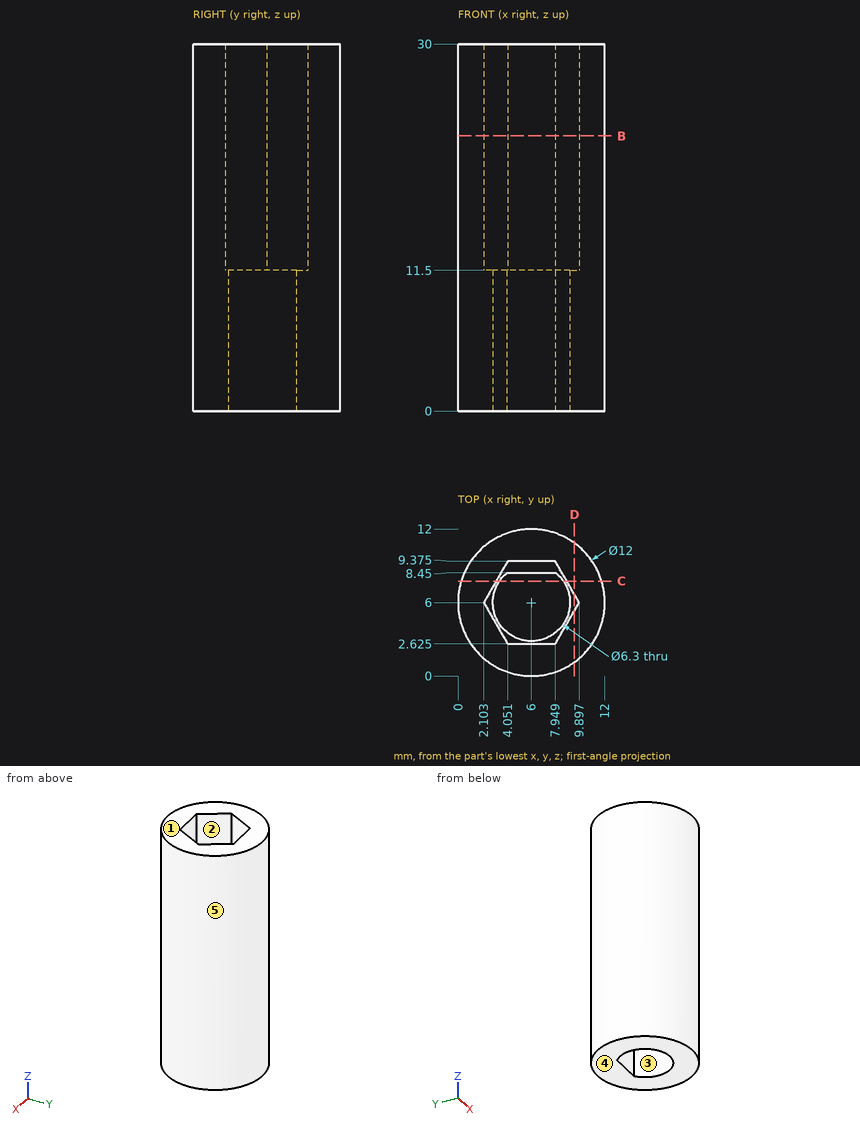
Verification items for this drawing (mm, ordinates from the low corner). A direction names the side the tool comes from. Coordinates: 2 decimals unless noted, no trailing zeros. Write each loop counter-clockwise with the first axis right and the second up, starting at its lowest first coordinate (ties: lowest second). Pieces come first, ordered by that corner, then holes. Notation, with made-up numbers: M -32,42.5 L -22,42.5 A23 cw -22,80.5 Z; hole C 68.5,54 d9. An arc over 180 degrees is marked long. Use CSV: the item, a comma, the result in double quotes.
Q1. Set-up check for the marked faces 1 and 2: record each of +Z, -Z, +X, -X, +Y, -Y from which the full face is reachable in a straight line by a thin tool's end or side.
Computed values:
face 1,"+Z, +X, -X, +Y, -Y"
face 2,"+Z"
Q2. Go/stop test with flat-tipped pins: P1, Ø4.5, axis at x = 5.5, z = 22, coming from the +Y side; P2, Ø5, axis at x = 10.5, z = 24.5, coming from the +Y side; P3, Ø1, axis at x = 3.5, z = 9.5, coming from the -Y side. Record where each tip stops, or that it passes through.
Computed values:
P1,"y = 12"
P2,"y = 11.66"
P3,"y = 0.34"
Q3. Section check B-B, the plane z = 22.5. Enter the section's corners in (x, y) (1 decimal).
Computed values:
outline,"C 6,6 d12; hole M 2.1,6 L 4.1,2.6 L 7.9,2.6 L 9.9,6 L 7.9,9.4 L 4.1,9.4 Z"
Q4. Section check C-C, the plane y = 7.75. Enter the section's corners in (x, z).
Computed values:
outline,"M 0.26,0 L 3.38,0 L 3.38,11.5 L 3.11,11.5 L 3.11,30 L 0.26,30 Z; M 8.62,0 L 11.74,0 L 11.74,30 L 8.89,30 L 8.89,11.5 L 8.62,11.5 Z"
Q5. Thickness scan on line 1 along Y through (x, z) = (6, 27.5) (1 decimal); line 2 along Y through (x, z) = (6, 6.5); line 3 along X through (y, z) = (7.75, 10.75). Record the ranges inside material, lowest first. Write a range as [from, to].
Computed values:
line 1,"[0, 2.6], [9.4, 12]"
line 2,"[0, 2.85], [8.45, 12]"
line 3,"[0.26, 3.38], [8.62, 11.74]"
Q6. Section check D-D, the plane x = 9.5. Enter the section's corners in (y, z), and give its area (3 significant figures).
Computed values:
outline,"M 1.13,0 L 10.87,0 L 10.87,30 L 6.69,30 L 6.69,11.5 L 5.31,11.5 L 5.31,30 L 1.13,30 Z"
area,"267 mm²"
Q7. Mould release check, pull along X, two halves, no side actions. Record for the marked faces 3, 4 and 5: pulls with the +X half, pulls with the -X half, needs draft (parallel to the pull), parting line crosses it, or undercut.
Computed values:
face 3,"undercut"
face 4,"needs draft"
face 5,"parting line crosses it"
